Verification items for the finished model (mm, model axes). A direction names the side the tool comes from. Coordinates: 2 decimals unless noted, no trailing zeros. Order: outer loops, then holes, each group sorted by start corner. A loop starts at its lowest first (then second) coordinate and runs counter-clockwise, first axis right, second up.
Q1. Depth check by flat-ended pin: P1, Ø6, axis at x = -7.5, z = -6.5, coming from the +Y side; P2, Ø6, axis at x = -53, z = 35.5, coming from the -Y side; P3, Ø12, axis at x = -78.5, z = 38.5, coming from the -Y side; P4, Ø2.5, axis at x = 0, z = 103.5, coming from the +Y side. Enter the tip coordinate at first touch or a pass-through.
Q2. Cross-section at A-A, the plane z = 0. Record the boundary of the cut face in (x, y), and give its area (3 significant figures).
Q3. Thickness scan on line 1 (Y direction, x = 58, z = -86.5); line 2 (Y direction, x = 81.5, z = -50.5). Record the ranges inside material, lowest first.
Q4. Set-up check for faces 1 (the flat face through (-96, 285.383, -31)), 2 (the cylindrical face through (-23.196, 284.13, -104.456)): record each of +Z, -Z, +X, -X, +Y, -Y from which the full face is reachable in a straight line by a thin tool's end or side.
Q5. Cross-section at B-B, the plane x = 37.5. Record the boundary of the cut face in (y, z), and give its area (3 significant figures).
from build123d import *

# Parameters (mm, degrees)
SKETCH4_R          = 1.4732
CUT_EXTRUDE1_DEPTH = 153.597454552


with BuildPart() as part:
    # Sketch1 one side → Revolve1 (revolve)
    with BuildSketch(Plane.XY):
        with BuildLine():
            ThreePointArc((100.434849632, 285.382712475), (50.944900471, 298.219832868), (0, 302.54))
            Line((0, 302.54), (0, 300))
            ThreePointArc((0, 300), (50.730593618, 295.679567896), (100, 282.842712475))
            Line((100, 282.842712475), (107, 282.842712475))
            Line((107, 282.842712475), (107, 285.382712475))
            Line((107, 285.382712475), (100.434849632, 285.382712475))
        make_face()
    revolve(axis=Axis((0, 282.842712475, 0), (0, -1, 0)))

    # Sketch4 → Cut-Extrude1 (cut, through all)
    with BuildSketch(Plane.XZ.offset(-282.842712475)):
        with Locations(Location((0, 103.5, 0), (0, 0, 270))):
            Circle(SKETCH4_R)
        with Locations(Location((89.633629292, 51.75, 0), (0, 0, 270))):
            Circle(SKETCH4_R)
        with Locations(Location((89.633629292, -51.75, 0), (0, 0, 270))):
            Circle(SKETCH4_R)
        with Locations(Location((0, -103.5, 0), (0, 0, 270))):
            Circle(SKETCH4_R)
        with Locations(Location((-89.633629292, -51.75, 0), (0, 0, 270))):
            Circle(SKETCH4_R)
        with Locations(Location((-89.633629292, 51.75, 0), (0, 0, 270))):
            Circle(SKETCH4_R)
    extrude(amount=-CUT_EXTRUDE1_DEPTH, mode=Mode.SUBTRACT)


solid = part.part
Check values:
1. P1: stops at y = 302.46
1. P2: stops at y = 292.47
1. P3: stops at y = 285.08
1. P4: passes through
2. outline: (-107, 282.84) - (-100, 282.84) arc R300 cw to (100, 282.84) - (107, 282.84) - (107, 285.38) - (100.43, 285.38) arc R302.54 ccw to (-100.43, 285.38) - (-107, 285.38) - close
2. area: 553 mm2
3. line 1: y = 282.84 to 285.38
3. line 2: y = 284.27 to 286.95
4. face 1: +Y
4. face 2: +Y, -Y
5. outline: (282.84, -100.21) - (285.38, -100.21) - (285.38, -93.17) arc R300.21 ccw to (285.38, 93.17) - (285.38, 100.21) - (282.84, 100.21) - (282.84, 92.7) arc R297.65 cw to (282.84, -92.7) - close
5. area: 521 mm2
